Check sheet for the modelled part. Datum: model origin and axes. Units: mm. A direction names the side the tool comes from. Give positions to 0.01 mm unless a question says otherwise; leave off trailing zeros. Order: outer loops, then holes, each group sorted by start corner. A loop starts at its lowest first (then second) coordinate and runs counter-clockwise, first axis right, second up. Notation, with made-up numbers: (67.25, 86) -> (91.25, 86) arc R21 ccw to (91.25, 124) -> close; hole circle Ø4 at (70.25, 41). An arc over 180 degrees is marked (long way). Answer in a Markdown table with one row per item. Add a question column.
(1) Set-up check for faces 1 (the face through (-0.1, -20.2, -139.5)), 2 (the face through (-21.46, 0.86, 72.92)): record each of +Z, -Z, +X, -X, +Y, -Y from which the full face is reachable in a straight line by a thin tool's end or side.
(2) Cross-section at A-A (y = -7). Record the cut outline in (x, z) (3 decimals), then the cut area to 3 significant figures.
(3) Thickness scan on L1, parallel to X at y = 0.5, z = -101; L2, parallel to Y at x = 0, z = 17; L3, parallel to X at y = -16, z = -25.5. Record the ranges inside material, lowest first. Write a range as [from, to].
(4) Go/stop test with flat-tipped pins: pin 1 (4 mm diameter, centred on x = 3.5, y = -16.5, fed in from -Z); pin 2 (6 mm diameter, centred on x = -13.5, z = 71.5, fed in from -Y); pin 3 (3.5 mm diameter, centred on y = 0, z = 75, fed in from -X); pin 4 (4 mm diameter, centred on x = 9, z = 96.5, fed in from -Y). Record where each tip stops, or that it passes through.
(5) Release check for a two-part mould opening along Y. For faces 3 (the face through (0.61, -22.99, -1.95)), 4 (the face through (-21.46, 0.86, -77.08)), 5 (the face through (-0.1, -20.2, 139.5)) record: released by +Y, released by -Y, zero draft, split by the parting line, or undercut.
(6) Cross-section at C-C (z = -50). Record the cut outline in (x, y) (3 decimals).
(7) Cross-section at B-B (x = 0). Record the cut outline in (y, z), then the cut area to 3 significant figures.
Autodesk Inventor part; units mm, degrees
ref_plane "YZ Plane" through (0, 0, 0) normal (1, 0, 0) x (0, 1, 0)
ref_plane "XZ Plane" through (0, 0, 0) normal (0, 1, 0) x (-1, 0, 0)
ref_plane "XY Plane" through (0, 0, 0) normal (0, 0, 1) x (1, 0, 0)
sketch "Sketch1" plane through (0, 0, 0) normal (0, 0, 1) x (1, 0, 0)
  circle A0 centre (0, 0) radius 20
  circle A1 centre (0, 0) radius 23
  dimension "d0" = 40
  dimension "d1" = 46
extrude "Extrusion1" add sketch "Sketch1" along normal mid plane 279
sketch "Sketch2" plane through (0, 0, 0) normal (1, 0, 0) x (0, 1, 0)
  line L0 (0, 105) -> (0, -105)
  line L1 (-105, 0) -> (105, 0)
  point P0 (0, 0)
  point P1 (0, 75)
  point P2 (0, -75)
  dimension "d19" = 75
  dimension "d20" = 150
hole "Hole1" at (0, 0, 75) at (0, 0, -75) direction (-1, 0, 0) diameter 4.5 end through all
sketch "Sketch3" plane through (0, 0, 0) normal (1, 0, 0) x (0, 1, 0)
  line L0 (23, -139.5) -> (7, -139.5)
  line L1 (7, -139.5) -> (7, 139.5)
  line L2 (7, 139.5) -> (23, 139.5)
  line L3 (23, 139.5) -> (23, -139.5)
  line L4 (23, 139.5) -> (-23, 139.5)
  line L5 (-23, -139.5) -> (23, -139.5)
  line L6 (0, 198.1) -> (0, -198.1)
  point P0 (0, 0)
  dimension "d13" = 0
  dimension "d14" = 0
  dimension "d15" = 7
extrude "Extrusion2" cut sketch "Sketch3" along normal through all both and the other way through all contours L0 L1 L2 L3
properties part number "Top_Tilt Pipe" material "PVC-Piping"
Answer below:
| question | item | result |
|---|---|---|
| 1 | face 1 | -Z, +X, -X, +Y, -Y |
| 1 | face 2 | -X |
| 2 | outline | (-21.909, -139.5) -> (-18.735, -139.5) -> (-18.735, 139.5) -> (-21.909, 139.5) -> close; (18.735, -139.5) -> (21.909, -139.5) -> (21.909, 139.5) -> (18.735, 139.5) -> close |
| 2 | area | 1,770 mm² |
| 3 | L1 | x = [-22.99, -19.99], [19.99, 22.99] |
| 3 | L2 | y = [-23, -20] |
| 3 | L3 | x = [-16.52, -12], [12, 16.52] |
| 4 | pin 1 | passes through |
| 4 | pin 2 | stops at y = -20.46 |
| 4 | pin 3 | stops at x = 19.92 |
| 4 | pin 4 | stops at y = -21.91 |
| 5 | face 3 | split by the parting line |
| 5 | face 4 | undercut |
| 5 | face 5 | zero draft |
| 6 | outline | (-21.909, 7) arc R23 ccw (long way) to (21.909, 7) -> (18.735, 7) arc R20 cw (long way) to (-18.735, 7) -> close |
| 7 | outline | (-23, -139.5) -> (-20, -139.5) -> (-20, 139.5) -> (-23, 139.5) -> close |
| 7 | area | 837 mm² |
